```python
from build123d import *

# Parameters (mm, degrees)
ESQUISSE1_R        = 11
BOSS_EXTRU_1_DEPTH = 49.9
ESQUISSE2_R        = 22
ESQUISSE2_R_2      = 2.6
BOSS_EXTRU_2_DEPTH = 2.4
BOSS_EXTRU_3_START = 5
ESQUISSE3_R        = 11
BOSS_EXTRU_3_DEPTH = 5
ESQUISSE4_R        = 3.9
BOSS_EXTRU_4_DEPTH = 9


with BuildPart() as part:
    # Esquisse1 → Boss.-Extru.1 (new body)
    with BuildSketch(Plane.XY):
        Circle(ESQUISSE1_R)
    extrude(amount=BOSS_EXTRU_1_DEPTH)

    # Esquisse2 → Boss.-Extru.2 (add)
    with BuildSketch(Plane(origin=(0, 0, 0), x_dir=(-1, 0, 0), z_dir=(0, 0, -1))):
        Circle(ESQUISSE2_R)
        with Locations((17.5, 0)):
            Circle(ESQUISSE2_R_2, mode=Mode.SUBTRACT)
        with Locations((-8.75, -15.155444566)):
            Circle(ESQUISSE2_R_2, mode=Mode.SUBTRACT)
        with Locations((-8.75, 15.155444566)):
            Circle(ESQUISSE2_R_2, mode=Mode.SUBTRACT)
    extrude(amount=BOSS_EXTRU_2_DEPTH)

    # Esquisse3 → Boss.-Extru.3 (add)
    with BuildSketch(Plane(origin=(0, 0, -2.4), x_dir=(-1, 0, 0), z_dir=(0, 0, -1)).offset(BOSS_EXTRU_3_START)):
        with Locations(Location((0, 0, 0), (0, 0, 180))):
            Circle(ESQUISSE3_R)
    extrude(amount=-BOSS_EXTRU_3_DEPTH)

    # Esquisse4 → Boss.-Extru.4 (add)
    with BuildSketch(Plane(origin=(0, 0, -7.4), x_dir=(-1, 0, 0), z_dir=(0, 0, -1))):
        Circle(ESQUISSE4_R)
    extrude(amount=BOSS_EXTRU_4_DEPTH)


solid = part.part
```
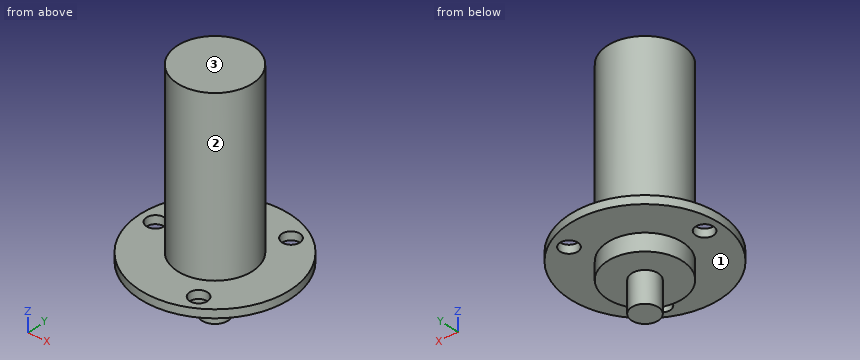
The listing builds one solid part. Answer for the finished solid, in the listing's coordinates (mm). Face numbers are marked on the shaded views. A direction names the side the tool comes from. Coordinates: 2 decimals unless noted, no trailing zeros. Write each loop counter-clockwise with the first axis right and the second up, starting at its lowest first coordinate (ties: lowest second). Pieces come first, ordered by that corner, then holes. Notation, with made-up numbers: (23.5, -3) - (59.5, -3) arc R19 ccw to (59.5, 32) - close; hole circle Ø3 at (45.25, 19). An arc over 180 degrees is marked (long way). Return JSON: item names as keys, results as strings. Group by question number.
1. Straight lines are drawn through the part: L1, parallel to Y at x = 8.75, z = -1; L2, parallel to Z at x = -16.5, y = -13.5; L3, parallel to Z at x = -6, y = 1.5. For each, find the intervals that lie inside material, in ascending order.
2. A cutting plane is placed at A-A, the plane x = 0. Determine the outline of the cut face in (y, z), plus the area to 3 significant figures.
3. Given pin 1 (1.5 mm diameter, centred on x = 17, y = -7, fed in from -Z); pin 2 (1 mm diameter, centred on y = 7.5, z = 42, fed in from -X); pin 3 (8.5 mm diameter, centred on x = 8.75, y = 15.16, fed in from +Z); pin 4 (22 mm diameter, centred on x = 10.5, y = -10, fed in from -Z), each flat-ended and moving along its own axis, determine where each tip first touches the part or whether it passes through.
4. A cutting plane is placed at B-B, the plane y = 13.5. Determine the outline of the cut face in (x, z), plus the area to 3 significant figures.
5. Which of the six approach directions +Z, -Z, +X, -X, +Y, -Y give full straight-line access (tool end or side, diameter ignored) to the marked faces 1, 2 and 3?
6. A cutting plane is placed at C-C, the plane x = 8.75. Determine the outline of the cut face in (y, z), plus the area to 3 significant figures.
7. A cutting plane is placed at D-D, the plane x = -17.5. Determine the outline of the cut face in (y, z), plus the area to 3 significant figures.
Ans:
{
 "1": {"L1": "-20.19 to -17.76, -12.56 to 12.56, 17.76 to 20.19", "L2": "-2.4 to 0", "L3": "-7.4 to 49.9"},
 "2": {"outline": "(-22, -2.4) - (-11, -2.4) - (-11, -7.4) - (-3.9, -7.4) - (-3.9, -16.4) - (3.9, -16.4) - (3.9, -7.4) - (11, -7.4) - (11, -2.4) - (22, -2.4) - (22, 0) - (11, 0) - (11, 49.9) - (-11, 49.9) - (-11, 0) - (-22, 0) - close", "area": "1,380 mm²"},
 "3": {"pin 1": "z = -2.4", "pin 2": "x = -8.49", "pin 3": "z = 0", "pin 4": "z = -16.4"},
 "4": {"outline": "(-17.37, -2.4) - (6.75, -2.4) - (6.75, 0) - (-17.37, 0) - close; (10.75, -2.4) - (17.37, -2.4) - (17.37, 0) - (10.75, 0) - close", "area": "73.8 mm²"},
 "5": {"face 1": "-Z", "face 2": "+Z", "face 3": "+Z, +X, -X, +Y, -Y"},
 "6": {"outline": "(-20.19, -2.4) - (-17.76, -2.4) - (-17.76, 0) - (-20.19, 0) - close; (-12.56, -2.4) - (-6.67, -2.4) - (-6.67, -7.4) - (6.67, -7.4) - (6.67, -2.4) - (12.56, -2.4) - (12.56, 0) - (6.67, 0) - (6.67, 49.9) - (-6.67, 49.9) - (-6.67, 0) - (-12.56, 0) - close; (17.76, -2.4) - (20.19, -2.4) - (20.19, 0) - (17.76, 0) - close", "area": "804 mm²"},
 "7": {"outline": "(-13.33, -2.4) - (-2.6, -2.4) - (-2.6, 0) - (-13.33, 0) - close; (2.6, -2.4) - (13.33, -2.4) - (13.33, 0) - (2.6, 0) - close", "area": "51.5 mm²"}
}
